from build123d import *

# Parameters (mm, degrees)
BOSS_EXTRUDE1_DEPTH     = 38.1
F_1_4_CLEARANCE_HOLE3_D = 6.7564


with BuildPart() as part:
    # Sketch1 → Boss-Extrude1 (new body)
    with BuildSketch(Plane(origin=(0, 0, 0), x_dir=(0, 0, -1), z_dir=(1, 0, 0))):
        Polygon((-69.85, 0), (69.85, 0), (69.85, 6.35), (12.7, 6.35), (12.7, 25.4), (6.35, 25.4), (6.35, 6.35), (-6.35, 6.35), (-6.35, 25.4), (-12.7, 25.4), (-12.7, 6.35), (-69.85, 6.35), align=None)
    extrude(amount=BOSS_EXTRUDE1_DEPTH)

    # 1/4 Clearance Hole3 (through all)
    with Locations(Plane.XY.offset(12.7)):
        with Locations((31.75, 13.5255)):
            Hole(F_1_4_CLEARANCE_HOLE3_D / 2)


solid = part.part
Check sheet for the modelled part. Datum: model origin and axes. Units: mm. A direction names the side the tool comes from. Coordinates: 2 decimals unless noted, no trailing zeros. Loops run counter-clockwise (first coordinate to the right, second up) from the corner with the lowest first, then second, coordinate; pieces in that order, holes last. Notation, with made-up numbers: (28, 38.5) -> (35, 38.5) arc R23 cw to (35, 71.5) -> close; hole circle Ø5 at (-23, 79). An arc over 180 degrees is marked (long way). Answer in a Markdown table with one row per item.
1. Sectioned sample at C-C, the plane x = 10.5. Record the boundary of the cut face in (y, z), then the cut area to 3 significant figures.
Check values:
| item | result |
|---|---|
| outline | (0, -69.85) -> (6.35, -69.85) -> (6.35, -12.7) -> (25.4, -12.7) -> (25.4, -6.35) -> (6.35, -6.35) -> (6.35, 6.35) -> (25.4, 6.35) -> (25.4, 12.7) -> (6.35, 12.7) -> (6.35, 69.85) -> (0, 69.85) -> close |
| area | 1,130 mm2 |
2. Access from +Z, -Z, +X, -X, +Y, -Y to the whole of each face (thin tool, end or side, straight path). Record for faces 1 (the face through (19, 6.35, 0)), 2 (the face through (28.63, 12.23, 9.48)), 3 (the face through (19, 6.35, -42)), 4 (the face through (19, 6.35, 41)).
Check values:
| item | result |
|---|---|
| face 1 | +X, -X, +Y |
| face 2 | +Z, -Z |
| face 3 | -Z, +X, -X, +Y |
| face 4 | +Z, +X, -X, +Y |
3. Sectioned sample at A-A, the plane y = 18.5. Record the boundary of the cut face in (x, z), then the cut area to 3 significant figures.
Check values:
| item | result |
|---|---|
| outline | (0, -12.7) -> (38.1, -12.7) -> (38.1, -6.35) -> (0, -6.35) -> close; (0, 6.35) -> (38.1, 6.35) -> (38.1, 12.7) -> (0, 12.7) -> close |
| area | 484 mm2 |
4. Go/stop test with flat-tipped pins: pin 1 (15 mm diameter, centred on x = 17, y = 16.5, fed in from +Z); pin 2 (8 mm diameter, centred on x = 7.5, y = 8, fed in from -Z); pin 3 (9 mm diameter, centred on x = 31.75, y = 13.53, fed in from -Z); pin 4 (5 mm diameter, centred on x = 32.5, z = -39, fed in from +Y). Record where each tip stops, or that it passes through.
Check values:
| item | result |
|---|---|
| pin 1 | stops at z = 12.7 |
| pin 2 | stops at z = -69.85 |
| pin 3 | stops at z = -12.7 |
| pin 4 | stops at y = 6.35 |
5. Material ranges on line 1 along Z through (x, y) = (10, 17.25); line 2 along Y through (x, z) = (31.75, -9); line 3 along Y through (x, z) = (16, -35), recorded low to high. Write a range as [from, to].
Check values:
| item | result |
|---|---|
| line 1 | z = [-12.7, -6.35], [6.35, 12.7] |
| line 2 | y = [0, 10.15], [16.9, 25.4] |
| line 3 | y = [0, 6.35] |
6. Sectioned sample at D-D, the plane z = 29.5. Record the boundary of the cut face in (x, y), then the cut area to 3 significant figures.
Check values:
| item | result |
|---|---|
| outline | (0, 0) -> (38.1, 0) -> (38.1, 6.35) -> (0, 6.35) -> close |
| area | 242 mm2 |
7. Sectioned sample at B-B, the plane x = 31.75. Record the boundary of the cut face in (y, z), then the cut area to 3 significant figures.
Check values:
| item | result |
|---|---|
| outline | (0, -69.85) -> (6.35, -69.85) -> (6.35, -12.7) -> (10.15, -12.7) -> (10.15, -6.35) -> (6.35, -6.35) -> (6.35, 6.35) -> (10.15, 6.35) -> (10.15, 12.7) -> (6.35, 12.7) -> (6.35, 69.85) -> (0, 69.85) -> close; (16.9, -12.7) -> (25.4, -12.7) -> (25.4, -6.35) -> (16.9, -6.35) -> close; (16.9, 6.35) -> (25.4, 6.35) -> (25.4, 12.7) -> (16.9, 12.7) -> close |
| area | 1,040 mm2 |
8. Release check for a two-part mould opening along Y. For faces 5 (the face through (19, 0, 1)), 6 (the face through (28.63, 12.23, -9.57)), 7 (the face through (19, 16, -12.7)) record: released by +Y, released by -Y, zero draft, split by the parting line, or undercut.
Check values:
| item | result |
|---|---|
| face 5 | released by -Y |
| face 6 | undercut |
| face 7 | zero draft |
